Here's how the part is built. I have some questions about the finished solid (model axes, mm). Face numbers are marked on the shaded views. Give positions to 0.01 mm unless a question says otherwise; leave off trailing zeros. Order: outer loops, then holes, each group sorted by start corner. A loop starts at its lowest first (then second) coordinate and runs counter-clockwise, first axis right, second up. Notation, with made-up numbers: (73, -8.75) -> (78, -8.75) arc R25 ccw to (78, 23.25) -> close; hole circle Ø3 at (20.5, 31.5). An arc over 180 degrees is marked (long way). Write each question's results on one line, items separated by ' | '. Start each with the question number.
Q1. I need wall thicknesses on line 1 along Y through (x, z) = (0.7, 0); line 2 along Z through (x, y) = (1.95, -24.5); line 3 along Y through (x, z) = (0.3, -90.5). Which ranges of each line are inside material? Lowest first, please. Write a range as [from, to].
Q2. Imagine slicing it at D-D, the plane x = 0.5. State how many separate pieces and enclosed holes the cut face has, then the cut area to 3 significant figures.
Q3. Imagine slicing it at B-B, the plane y = 8. Please give me the cut outline in (x, z).
Q4. Thinking about a two-plate mould opening in X: for the marked faces 1 and 2, which applies, pulls with the +X half, pulls with the -X half, needs draft (parallel to the pull), parting line crosses it, or undercut?
Q5. I'm going to push flat-ended pins straight in: pin 1 (0.6 mm diameter, centred on x = 1, z = -65.5, fed in from +Y); pin 2 (1 mm diameter, centred on x = 1.5, z = -2.5, fed in from -Y); pin 3 (0.6 mm diameter, centred on x = 0.5, z = -139, fed in from +Y). Where does each tip first touch, or does it pass through?
Q6. Imagine slicing it at C-C, the plane z = -31.5. Please give me the cut outline in (x, y), then the cut area to 3 significant figures.
Q7. Imagine slicing it at A-A, the plane z = 0. Please give me the cut outline in (x, y), then the cut area to 3 significant figures.
```python
from build123d import *

# Parameters (mm, degrees)
SKETCH_1_W      = 15
SKETCH_1_H      = 2.5
SKETCH_1_R      = 1.55
EXTRUDE_1_DEPTH = 2
FILLET_1_R      = 1


with BuildPart() as part:
    # 草图1 → 凸台-拉伸1 (new body)
    with BuildSketch(Plane(origin=(0, 0, 0), x_dir=(0, 0, -1), z_dir=(1, 0, 0))):
        Polygon((7.5, 12), (-7.5, 12), (-7.5, -4), (15.739132695, -4), (59.924651317, -30.703841765), (61.202132807, -30), (63.924651317, -28.5), (90.154353452, -46.86623516), (118.807980924, -37), (132.770523856, -37), (153.1, -30), (153.1, -21.5), (93.1, -19.40475383), align=None)
        with Locations((128, -30.75)):
            Rectangle(SKETCH_1_W, SKETCH_1_H, mode=Mode.SUBTRACT)
        with Locations((107, -30.75)):
            Rectangle(SKETCH_1_W, SKETCH_1_H, mode=Mode.SUBTRACT)
        with Locations((86, -30.75)):
            Rectangle(SKETCH_1_W, SKETCH_1_H, mode=Mode.SUBTRACT)
        with BuildLine():
            Line((86, -26.65), (74, -26.65))
            ThreePointArc((74, -26.65), (72.95, -27.7), (71.9, -26.65))
            Line((71.9, -26.65), (71.9, -24.35))
            ThreePointArc((71.9, -24.35), (72.95, -23.3), (74, -24.35))
            Line((74, -24.35), (86, -24.35))
            ThreePointArc((86, -24.35), (87.05, -23.3), (88.1, -24.35))
            Line((88.1, -24.35), (88.1, -26.65))
            ThreePointArc((88.1, -26.65), (87.05, -27.7), (86, -26.65))
        make_face(mode=Mode.SUBTRACT)
        with BuildLine():
            Line((146, -26.65), (134, -26.65))
            ThreePointArc((134, -26.65), (132.95, -27.7), (131.9, -26.65))
            Line((131.9, -26.65), (131.9, -24.35))
            ThreePointArc((131.9, -24.35), (132.95, -23.3), (134, -24.35))
            Line((134, -24.35), (146, -24.35))
            ThreePointArc((146, -24.35), (147.05, -23.3), (148.1, -24.35))
            Line((148.1, -24.35), (148.1, -26.65))
            ThreePointArc((148.1, -26.65), (147.05, -27.7), (146, -26.65))
        make_face(mode=Mode.SUBTRACT)
        Polygon((54.105215944, -20.5), (7, 6.857560085), (81.568555955, -20.5), align=None, mode=Mode.SUBTRACT)
        Circle(SKETCH_1_R, mode=Mode.SUBTRACT)
        with Locations((0, 8)):
            Circle(SKETCH_1_R, mode=Mode.SUBTRACT)
        Polygon((79.681548741, -34.65), (113.34666254, -34.65), (90.779143943, -42.420619816), align=None, mode=Mode.SUBTRACT)
    extrude(amount=EXTRUDE_1_DEPTH)

    # 圆角1
    fillet_1_edges = [part.edges().sort_by_distance(p)[0] for p in [
        (1, -32, -135.5),
        (1, -29.5, -135.5),
        (1, -29.5, -120.5),
        (1, -32, -120.5),
        (1, -32, -114.5),
        (1, -29.5, -114.5),
        (1, -29.5, -99.5),
        (1, -32, -99.5),
        (1, -32, -93.5),
        (1, -29.5, -93.5),
        (1, -29.5, -78.5),
        (1, -32, -78.5),
        (1, -34.65, -113.34666254),
        (1, -34.65, -79.681548741),
        (1, -42.420619816, -90.779143943),
        (1, 6.857560085, -7),
        (1, -20.5, -54.105215944),
        (1, -20.5, -81.568555955),
        (1, -46.86623516, -90.154353452),
        (1, -28.5, -63.924651317),
        (1, -30.703841765, -59.924651317),
        (1, -4, -15.739132695),
        (1, -4, 7.5),
        (1, 12, 7.5),
        (1, 12, -7.5),
        (1, -19.40475383, -93.1),
        (1, -21.5, -153.1),
        (1, -30, -153.1),
        (1, -37, -132.770523856),
        (1, -37, -118.807980924),
    ]]
    fillet(fillet_1_edges, radius=FILLET_1_R)


solid = part.part
```
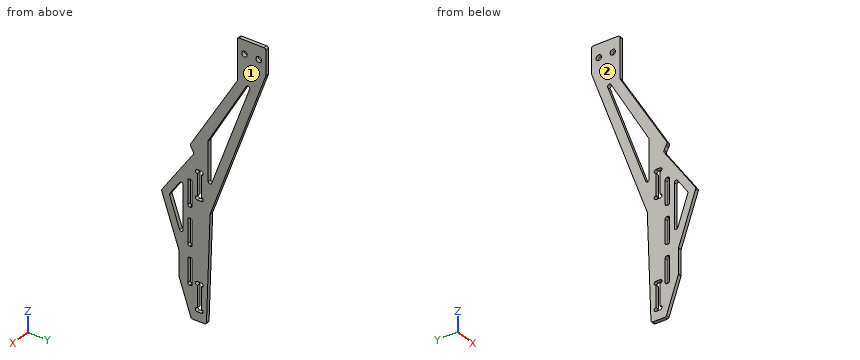
Geometry check:
1) line 1: [-4, -1.55], [1.55, 6.45], [9.55, 12] | line 2: [-153.1, -148.1], [-131.9, -88.1], [-71.9, -49.66] | line 3: [-46.74, -42.21], [-34.65, -32], [-29.5, -18.45]
2) separate pieces: 1 | enclosed holes: 9 | area: 2,300 mm²
3) outline: (0, -18.4) -> (2, -18.4) -> (2, -1.55) -> (0, -1.55) -> close; (0, 1.55) -> (2, 1.55) -> (2, 7.5) -> (0, 7.5) -> close
4) face 1: pulls with the +X half | face 2: pulls with the -X half
5) pin 1: y = -9.17 | pin 2: y = -4 | pin 3: y = -21
6) outline: (0, -13.53) -> (2, -13.53) -> (2, -7.37) -> (0, -7.37) -> close; (0, -2.13) -> (2, -2.13) -> (2, 3.19) -> (0, 3.19) -> close | area: 23.0 mm²
7) outline: (0, -4) -> (2, -4) -> (2, -1.55) -> (0, -1.55) -> close; (0, 1.55) -> (2, 1.55) -> (2, 6.45) -> (0, 6.45) -> close; (0, 9.55) -> (2, 9.55) -> (2, 12) -> (0, 12) -> close | area: 19.6 mm²
